Design review of the part built by this model. Coordinates are the model's own, in mm. A direction names the side the tool comes from. Give positions to 0.01 mm unless a question says otherwise; leave off trailing zeros. Write each loop counter-clockwise with the first axis right and the second up, starting at its lowest first coordinate (ties: lowest second). Pieces come first, ordered by that corner, then holes. Notation, with made-up numbers: (-21, -9) -> (5, -9) arc R14 ccw to (5, 9) -> close; hole circle Ø9 at (44, 39.25). An arc over 180 degrees is marked (long way). Return JSON: item names as keys, results as strings. Group by question number.
from build123d import *

# Parameters (mm, degrees)
SKETCH1_W            = 355
SKETCH1_H            = 6.35
BOSS_EXTRUDE1_DEPTH  = 200
SKETCH28_R           = 1.75
RELIEF_CUTS_DEPTH    = 10
M5_CLEARANCE_HOLE1_D = 5.8
BOSS_EXTRUDE2_DEPTH  = 6.35


with BuildPart() as part:
    # Sketch1 → Boss-Extrude1 (new, symmetric)
    with BuildSketch(Plane(origin=(0, 0, 0), x_dir=(0, 0, -1), z_dir=(1, 0, 0))):
        with Locations((0, -3.175)):
            Rectangle(SKETCH1_W, SKETCH1_H)
    extrude(amount=BOSS_EXTRUDE1_DEPTH, both=True)

    # Sketch28 → Relief Cuts (cut)
    with BuildSketch(Plane(origin=(0, 0, 0), x_dir=(-1, 0, 0), z_dir=(0, 1, 0))):
        with Locations(Location((15, 111, 0), (0, 0, 90))):
            Circle(SKETCH28_R)
        with Locations(Location((15, 58, 0), (0, 0, 90))):
            Circle(SKETCH28_R)
        with Locations(Location((-10, 58, 0), (0, 0, 90))):
            Circle(SKETCH28_R)
        with Locations(Location((162.5, 68, 0), (0, 0, 90))):
            Circle(SKETCH28_R)
        with Locations(Location((177.5, 68, 0), (0, 0, 90))):
            Circle(SKETCH28_R)
        with BuildLine():
            Line((10, 62), (-5, 62))
            ThreePointArc((-5, 62), (-12.071067812, 64.928932188), (-15, 72))
            Line((-15, 72), (-15, 97))
            ThreePointArc((-15, 97), (-12.071067812, 104.071067812), (-5, 107))
            Line((-5, 107), (10, 107))
            ThreePointArc((10, 107), (17.071067812, 104.071067812), (20, 97))
            Line((20, 97), (20, 72))
            ThreePointArc((20, 72), (17.071067812, 64.928932188), (10, 62))
        make_face()
        with BuildLine():
            Line((168, 107), (172, 107))
            ThreePointArc((172, 107), (179.071067812, 104.071067812), (182, 97))
            Line((182, 97), (182, 82))
            ThreePointArc((182, 82), (179.071067812, 74.928932188), (172, 72))
            Line((172, 72), (168, 72))
            ThreePointArc((168, 72), (160.928932188, 74.928932188), (158, 82))
            Line((158, 82), (158, 97))
            ThreePointArc((158, 97), (160.928932188, 104.071067812), (168, 107))
        make_face()
    extrude(amount=-RELIEF_CUTS_DEPTH, mode=Mode.SUBTRACT)

    # M5 Clearance Hole1 (through all)
    with Locations(Plane(origin=(0, 0, 0), x_dir=(1, 0, 0), z_dir=(0, 1, 0))):
        with Locations((-119.5, 56), (-94.5, 56), (-94.5, -56), (-119.5, -56), (157, -68), (157, -14.5), (157, 43), (177, 43), (177, -68)):
            Hole(M5_CLEARANCE_HOLE1_D / 2)

    # Sketch33 → Boss-Extrude2 (add)
    with BuildSketch(Plane(origin=(0, 0, 0), x_dir=(1, 0, 0), z_dir=(0, 1, 0))):
        Polygon((200, 177.5), (200, -177.5), (316.322865072, -84.817675973), (316.322865072, 84.817675973), align=None)
    extrude(amount=-BOSS_EXTRUDE2_DEPTH)


solid = part.part
Q1. For L1, parallel to Z at x = -94.5, y = -5; L2, parallel to Z at x = 157, y = -2.75; L3, parallel to X at y = -3, z = -43, list the stretches that pass through material, from the lowest coordinate up. Write a range as from..to.
Q2. Take a section at B-B, the plane x = 240. Give the boundary of the cut face in (y, z), plus the area to 3 significant figures.
Q3. Insertion check: pin 1 (3.5 mm diameter, centred on x = 157, z = 14.5, fed in from -Y); pin 2 (3 mm diameter, centred on x = 210.5, y = -1, fed in from +Z). Each pin has a flat end and moves straight along its axis. Give the tip position at first contact, or say it passes through.
Q4. Mouldability with a two-part tool opening along X and no side actions: class faces 3 (the face through (257.347, -3.131, 131.808)), 4 (the face through (55, 0, -2)), 5 (the face through (-16.99, -3.13, 104.15)) as +X half, -X half, draft (parallel to the pull), parting line (faces both ways), or undercut.
Q5. Tool access review of faces 1 (the face through (55, -6.35, -2)), 2 (the face through (-17.15, -3.13, 65.01)): name each direction out of +Z, -Z, +X, -X, +Y, -Y from which nothing blocks a thin tool from reaching the whole face with its end or side.
Q6. Take a section at A-A, the plane y = -2. Count the separate pieces of the cut face and the enclosed holes in it, plus the area to 3 significant figures.
Final values:
{
 "1": {"L1": "z = -177.5..-58.9, -53.1..53.1, 58.9..177.5", "L2": "z = -177.5..-45.9, -40.1..11.6, 17.4..65.1, 70.9..177.5", "L3": "x = -200..154.1, 159.9..174.1, 179.9..316.32"},
 "2": {"outline": "(-6.35, -145.63) -> (0, -145.63) -> (0, 145.63) -> (-6.35, 145.63) -> close", "area": "1,850 mm²"},
 "3": {"pin 1": "passes through", "pin 2": "stops at z = 170.33"},
 "4": {"face 3": "+X half", "face 4": "draft", "face 5": "undercut"},
 "5": {"face 1": "+Z, -Z, +X, -X, -Y", "face 2": "+Y, -Y"},
 "6": {"separate pieces": "1", "enclosed holes": "16", "area": "170,000 mm²"}
}
